Autodesk Inventor part; units mm, degrees
ref_plane "YZ Plane" through (0, 0, 0) normal (1, 0, 0) x (0, 1, 0)
ref_plane "XZ Plane" through (0, 0, 0) normal (0, 1, 0) x (-1, 0, 0)
ref_plane "XY Plane" through (0, 0, 0) normal (0, 0, 1) x (1, 0, 0)
sketch "Boceto1" plane through (0, 0, 0) normal (0, 1, 0) x (-1, 0, 0)
  circle A0 centre (10.9374, 23.9581) radius 3
  point P0 (0, 0)
  dimension "d0" = 6
extrude "Extrusión1" add sketch "Boceto1" along normal blind 6
sketch "Boceto2" plane through (-10.9374, 6, 23.9581) normal (0, 1, 0) x (1, 0, 0)
  line L0 (0, 1.58) -> (1.3683, 0.79)
  line L1 (1.3683, 0.79) -> (1.3683, -0.79)
  line L2 (1.3683, -0.79) -> (0, -1.58)
  line L3 (0, -1.58) -> (-1.3683, -0.79)
  line L4 (-1.3683, -0.79) -> (-1.3683, 0.79)
  line L5 (-1.3683, 0.79) -> (0, 1.58)
  circle A0 centre (0, 0) radius 3
  line L6 (-3, 0) -> (0, 0)
  point P0 (10.9374, 23.9581)
  dimension "d11" = 1.58
  dimension "d12" = 1.58
extrude "Extrusión2" cut sketch "Boceto2" against normal blind 1.2 contours L0 L1 L2 L3 L4 L5
thread "Thread2"
chamfer "Chamfer1" distance 0.2 angle 45 1 edges at (-7.9374, 6, 23.9581)
properties part number "Tornillo Allen gusano M6 para Motor"
Read the model definition and answer for the solid it produces. Units are mm, in the model's axes. A direction names the side the tool comes from. Round coordinates to 2 decimals unless told otherwise and drop trailing zeros. Order: outer loops, then holes, each group sorted by start corner. A loop starts at its lowest first (then second) coordinate and runs counter-clockwise, first axis right, second up.
1) Flat-ended cylindrical pins translate along their axes: pin 1 (1 mm diameter, centred on y = 3.5, z = 26, fed in from +X); pin 2 (1.4 mm diameter, centred on x = -11, z = 24.5, fed in from +Y). Find the tip coordinate at first contact, or state that the pin passes through.
2) For faces 1 (the face through (-10.26, 5.41, 22.77)), 2 (the face through (-11, 0, 24)), determine the directions among +Z, -Z, +X, -X, +Y, -Y from which every point of the face is accessible in a straight line to the end or side of a thin tool.
3) Straight lines are drawn through the part: L1, parallel to Y at x = -10.4, z = 23.15; L2, parallel to Z at x = -8.45, y = 4.5; L3, parallel to Z at x = -10.1, y = 2.25. For each, find the intervals that lie inside material, in ascending order.
4) The mould has two halves that part along Z. Classify faces 3 (the face through (-12.1, 6, 22.8)), 4 (the face through (-8.557, 2.859, 25.784)), 5 (the face through (-11, 4.8, 24)): released by +Z, released by -Z, zero draft, split by the parting line, or undercut.
5) The part is cut by section A-A on y = 5. Write down the section's boundary in (x, z).
6) The part is cut by section B-B on y = 2.5. Write down the section's boundary in (x, z).
Resolved:
1. pin 1: stops at x = -8.36
1. pin 2: stops at y = 4.8
2. face 1: +Y
2. face 2: +Z, -Z, +X, -X, -Y
3. L1: y = 0 to 4.8
3. L2: z = 22.28 to 25.64
3. L3: z = 21.08 to 26.84
4. face 3: zero draft
4. face 4: split by the parting line
4. face 5: undercut
5. outline: circle Ø6 at (-10.94, 23.96); hole (-12.31, 23.17) - (-10.94, 22.38) - (-9.57, 23.17) - (-9.57, 24.75) - (-10.94, 25.54) - (-12.31, 24.75) - close
6. outline: circle Ø6 at (-10.94, 23.96)
